```python
from build123d import *

# Parameters (mm, degrees)
SKETCH_1_R      = 1.498311188
SKETCH_1_R_2    = 0.75
EXTRUDE_1_DEPTH = 1
SKETCH_3_W      = 1.886758636
SKETCH_3_H      = 2.158643663
SKETCH_3_W_2    = 2.358039665
SKETCH_3_H_2    = 1.729620016
EXTRUDE_2_DEPTH = 1


with BuildPart() as part:
    # 草图1 → 凸台-拉伸1 (new body)
    with BuildSketch(Plane.XY):
        with BuildLine():
            Line((-10.25, 2.25), (-8.3, 2.25))
            Line((-8.3, 2.25), (-8.3, 5.35))
            Line((-8.3, 5.35), (8.3, 5.35))
            Line((8.3, 5.35), (8.3, 2.25))
            Line((8.3, 2.25), (10.25, 2.25))
            ThreePointArc((10.25, 2.25), (12.5, 0), (10.25, -2.25))
            Line((10.25, -2.25), (8.3, -2.25))
            Line((8.3, -2.25), (8.3, -5.35))
            Line((8.3, -5.35), (-8.3, -5.35))
            Line((-8.3, -5.35), (-8.3, -2.25))
            Line((-8.3, -2.25), (-10.25, -2.25))
            ThreePointArc((-10.25, -2.25), (-12.5, 0), (-10.25, 2.25))
        make_face()
        with Locations((-10.25, 0)):
            Circle(SKETCH_1_R, mode=Mode.SUBTRACT)
        with Locations(Location((10.25, 0, 0), (0, 0, 180))):
            Circle(SKETCH_1_R, mode=Mode.SUBTRACT)
        with Locations((-6.35, -3.35)):
            Circle(SKETCH_1_R_2, mode=Mode.SUBTRACT)
        with Locations((-3.81, -3.35)):
            Circle(SKETCH_1_R_2, mode=Mode.SUBTRACT)
        with Locations((-1.27, -3.35)):
            Circle(SKETCH_1_R_2, mode=Mode.SUBTRACT)
        with Locations((1.27, -3.35)):
            Circle(SKETCH_1_R_2, mode=Mode.SUBTRACT)
        with Locations((3.81, -3.35)):
            Circle(SKETCH_1_R_2, mode=Mode.SUBTRACT)
        with Locations((6.35, -3.35)):
            Circle(SKETCH_1_R_2, mode=Mode.SUBTRACT)
    extrude(amount=EXTRUDE_1_DEPTH)

    # 草图3 → 凸台-拉伸2 (add)
    with BuildSketch(Plane(origin=(0, 0, 0), x_dir=(-1, 0, 0), z_dir=(0, 0, -1))):
        with Locations((-0.28460322, 0.170508759)):
            Rectangle(SKETCH_3_W, SKETCH_3_H)
        with Locations((5.064207673, 1.540607703)):
            Rectangle(SKETCH_3_W_2, SKETCH_3_H_2)
    extrude(amount=EXTRUDE_2_DEPTH)


solid = part.part
```
Design review of the part built by this model. Coordinates are the model's own, in mm. A direction names the side the tool comes from. Round coordinates to 2 decimals unless told otherwise and drop trailing zeros. Write each loop counter-clockwise with the first axis right and the second up, starting at its lowest first coordinate (ties: lowest second). Pieces come first, ordered by that corner, then holes.
Item 1: We need section B-B on y = -3.35. Write out the cut boundary in (x, z), and give its area (3 significant figures).
Item 2: Clearance check with flat-ended pins moving along their axes: pin 1 Ø1.1 at (y, z) = (4, 0.5) entering from -X; pin 2 Ø1.4 at (x, y) = (-3.81, -3.35) entering from -Z; pin 3 Ø0.5 at (x, z) = (0.5, -0.5) entering from +Y; pin 4 Ø0.8 at (x, z) = (9.5, 0.5) entering from +Y. State where each tip first meets the part, or that it passes through.
Item 3: The part is to be moulded in two halves that separate along Y. For faces 1 (the cylindrical face through (3.712, -2.606, 0.493)), 2 (the cylindrical face through (6.753, -2.718, 0.493)), 3 (the flat face through (-0.1, 5.35, 0.5)), 4 (the cylindrical face through (-12.5, 0, 0.5)), say which applies: +Y half, -Y half, draft (parallel to the pull), parting line (faces both ways), or undercut.
Item 4: For faces 5 (the flat face through (8.3, 3.8, 0.5)), 6 (the flat face through (9.3, -2.25, 0.5)), 7 (the flat face through (-3.885, 1.5, -0.5)), 8 (the flat face through (0.3, 1.25, -0.5)), list the 3-axis set-ups (+Z, -Z, +X, -X, +Y, -Y) from which the entire face can be reached by the end or side of a thin tool; tool diameter is ignored.
Item 5: For probe 1 along Y at (x, z) = (10.25, 0.5); probe 2 along Y at (x, z) = (-6.35, 0.45); probe 3 along X at (y, z) = (0.75, -0.25), list the stretches that pass through material, from the lowest coordinate up.
Item 6: We need section A-A on x = 3.81. Write out the cut boundary in (y, z).
Item 7: We need section C-C on y = 0. Write out the cut boundary in (x, z), and give its area (3 significant figures).
Item 8: We need section D-D on z = -0.6. Write out the cut boundary in (x, y).
Returned:
1. outline: (-8.3, 0) - (-7.1, 0) - (-7.1, 1) - (-8.3, 1) - close; (-5.6, 0) - (-4.56, 0) - (-4.56, 1) - (-5.6, 1) - close; (-3.06, 0) - (-2.02, 0) - (-2.02, 1) - (-3.06, 1) - close; (-0.52, 0) - (0.52, 0) - (0.52, 1) - (-0.52, 1) - close; (2.02, 0) - (3.06, 0) - (3.06, 1) - (2.02, 1) - close; (4.56, 0) - (5.6, 0) - (5.6, 1) - (4.56, 1) - close; (7.1, 0) - (8.3, 0) - (8.3, 1) - (7.1, 1) - close
1. area: 7.60 mm2
2. pin 1: stops at x = -8.3
2. pin 2: passes through
2. pin 3: stops at y = 1.25
2. pin 4: stops at y = 2.25
3. face 1: undercut
3. face 2: undercut
3. face 3: +Y half
3. face 4: parting line
4. face 5: +Z, -Z, +X, +Y
4. face 6: +Z, -Z, +X, -Y
4. face 7: -Z, +Y, -Y
4. face 8: -Z, +X, +Y
5. probe 1: y = -2.25 to -1.5, 1.5 to 2.25
5. probe 2: y = -5.35 to -4.1, -2.6 to 5.35
5. probe 3: x = -6.24 to -3.89, -0.66 to 1.23
6. outline: (-5.35, 0) - (-4.1, 0) - (-4.1, 1) - (-5.35, 1) - close; (-2.6, 0) - (5.35, 0) - (5.35, 1) - (-2.6, 1) - close
7. outline: (-12.5, 0) - (-11.75, 0) - (-11.75, 1) - (-12.5, 1) - close; (-8.75, 0) - (-0.66, 0) - (-0.66, -1) - (1.23, -1) - (1.23, 0) - (8.75, 0) - (8.75, 1) - (-8.75, 1) - close; (11.75, 0) - (12.5, 0) - (12.5, 1) - (11.75, 1) - close
7. area: 20.9 mm2
8. outline: (-6.24, 0.68) - (-3.89, 0.68) - (-3.89, 2.41) - (-6.24, 2.41) - close; (-0.66, -0.91) - (1.23, -0.91) - (1.23, 1.25) - (-0.66, 1.25) - close
